Geometry: final body of the model. Coordinates: model frame, mm. A direction names the side the tool comes from. Give positions to 0.01 mm unless a question says otherwise; leave off trailing zeros. Write each loop counter-clockwise with the first axis right and the second up, starting at its lowest first coordinate (ties: lowest second). Pieces come first, ordered by that corner, then holes.
Q1. Section A-A (y = 38.5). Return the cut outline in (x, z), plus the area to 3 significant figures.
Q2. Section D-D (x = 96). Return the cut outline in (y, z), plus the area to 3 significant figures.
Q3. Section C-C (z = 14.75). Return the cut outline in (x, y), plus the area to 3 significant figures.
Q4. Mould query, pull axis X, two halves, no side actions, for faces 1 (the cylindrical face through (114, 4.57, 14.62)), 2 (the flat face through (1, 34, 7)). Classes: +X half, -X half, draft (parallel to the pull), parting line (faces both ways), or undercut.
Q5. Line query: line 1 (Y direction, x = 57, z = 6.2); line 2 (X direction, y = 53.5, z = 17.5); line 3 (Y direction, x = 19.5, z = 6.25). Output: solid intervals per line, ascending.
Q6. Section B-B (x = 115.5). Return the cut outline in (y, z).
Q7. Reachability of faces 3 (the cylindrical face through (5.306, 76.765, 14.619)), 4 (the flat face through (3, 74, 6)), 5 (the flat face through (57, 53, 3)) from +Z, -Z, +X, -X, +Y, -Y: full face, straight path, thin tool, end or side. Return the list, or none.
Q8. Pin query (flat end, axial travel): pin 1 Ø5 at (x, y) = (89, 65.5) entering from +Z. Return the tip coordinate at first contact, or that it passes through.
from build123d import *

# Parameters (mm, degrees)
ESQUISSE1_W             = 120
ESQUISSE1_H             = 80
BOSS_EXTRU_1_DEPTH      = 3
ESQUISSE4_W             = 120
ESQUISSE4_H             = 80
ESQUISSE4_W_2           = 114
ESQUISSE4_H_2           = 74
BOSS_EXTRU_3_DEPTH      = 20
CONG_1_R                = 15
ESQUISSE5_R             = 1.5
ENL_V_MAT_EXTRU_1_DEPTH = 147.044513762
ESQUISSE7_R             = 3
ENL_V_MAT_EXTRU_3_DEPTH = 6
ESQUISSE8_W             = 6
ESQUISSE8_H             = 6
ESQUISSE8_R             = 1.5
BOSS_EXTRU_4_DEPTH      = 5
ENL_V_MAT_EXTRU_4_REACH = 148.045
ESQUISSE9_W             = 7
ESQUISSE9_H             = 12
CONG_3_R                = 1


with BuildPart() as part:
    # Esquisse1 → Boss.-Extru.1 (new body)
    with BuildSketch(Plane.XY):
        with Locations((60, 40)):
            Rectangle(ESQUISSE1_W, ESQUISSE1_H)
    extrude(amount=BOSS_EXTRU_1_DEPTH)

    # Esquisse4 → Boss.-Extru.3 (add)
    with BuildSketch(Plane.XY.offset(3)):
        with Locations((60, 40)):
            Rectangle(ESQUISSE4_W, ESQUISSE4_H)
        with Locations((60, 40)):
            Rectangle(ESQUISSE4_W_2, ESQUISSE4_H_2, mode=Mode.SUBTRACT)
    extrude(amount=BOSS_EXTRU_3_DEPTH)

    # Congé1
    cong_1_edges = [part.edges().sort_by_distance(p)[0] for p in [
        (3, 3, 13),
        (117, 3, 13),
        (117, 77, 13),
        (3, 77, 13),
    ]]
    fillet(cong_1_edges, radius=CONG_1_R)

    # Esquisse5 → Enlèv. mat.-Extru.1 (cut, through all)
    with BuildSketch(Plane.XY.offset(23)):
        with Locations((4.5, 75.5)):
            Circle(ESQUISSE5_R)
        with Locations((115.5, 75.5)):
            Circle(ESQUISSE5_R)
        with Locations((115.5, 4.5)):
            Circle(ESQUISSE5_R)
        with Locations((4.5, 4.5)):
            Circle(ESQUISSE5_R)
    extrude(amount=-ENL_V_MAT_EXTRU_1_DEPTH, mode=Mode.SUBTRACT)

    # Esquisse7 → Enlèv. mat.-Extru.3 (cut)
    with BuildSketch(Plane(origin=(0, 0, 0), x_dir=(-1, 0, 0), z_dir=(0, 0, -1))):
        with Locations((-115.5, 75.5)):
            Circle(ESQUISSE7_R)
        with Locations((-4.5, 75.5)):
            Circle(ESQUISSE7_R)
        with Locations((-4.5, 4.5)):
            Circle(ESQUISSE7_R)
        with Locations((-115.5, 4.5)):
            Circle(ESQUISSE7_R)
    extrude(amount=-ENL_V_MAT_EXTRU_3_DEPTH, mode=Mode.SUBTRACT)

    # Esquisse8 → Boss.-Extru.4 (add)
    # profile 1 of 4: a face of its own
    with BuildSketch(Plane.XY.offset(3)):
        with Locations((6, 52.5)):
            Rectangle(ESQUISSE8_W, ESQUISSE8_H)
        with Locations((6, 52.5)):
            Circle(ESQUISSE8_R, mode=Mode.SUBTRACT)
    # profile 2 of 4: a face of its own
    with BuildSketch(Plane.XY.offset(3)):
        with Locations((57, 52.5)):
            Rectangle(ESQUISSE8_W, ESQUISSE8_H)
        with Locations((57, 52.5)):
            Circle(ESQUISSE8_R, mode=Mode.SUBTRACT)
    # profile 3 of 4: a face of its own
    with BuildSketch(Plane.XY.offset(3)):
        with Locations((57, 27.5)):
            Rectangle(ESQUISSE8_W, ESQUISSE8_H)
        with Locations((57, 27.5)):
            Circle(ESQUISSE8_R, mode=Mode.SUBTRACT)
    # profile 4 of 4: a face of its own
    with BuildSketch(Plane.XY.offset(3)):
        with Locations((6, 27.5)):
            Rectangle(ESQUISSE8_W, ESQUISSE8_H)
        with Locations((6, 27.5)):
            Circle(ESQUISSE8_R, mode=Mode.SUBTRACT)
    extrude(amount=BOSS_EXTRU_4_DEPTH)

    # Esquisse9 → Enlèv. mat.-Extru.4 (cut, up to next)
    with BuildSketch(Plane.ZY, mode=Mode.PRIVATE) as enl_v_mat_extru_4_sk1:
        with Locations((7, 40)):
            Rectangle(ESQUISSE9_W, ESQUISSE9_H)
    enl_v_mat_extru_4_tool1 = extrude(enl_v_mat_extru_4_sk1.sketch, amount=-ENL_V_MAT_EXTRU_4_REACH, mode=Mode.PRIVATE) & part.part
    add(enl_v_mat_extru_4_tool1.solids().sort_by_distance((0, 40, 7))[0], mode=Mode.SUBTRACT)

    # Congé3
    cong_3_edges = [part.edges().sort_by_distance(p)[0] for p in [
        (60, 80, 0),
        (120, 40, 0),
        (60, 0, 0),
        (0, 80, 11.5),
        (120, 80, 11.5),
        (120, 0, 11.5),
        (0, 0, 11.5),
    ]]
    fillet(cong_3_edges, radius=CONG_3_R)


solid = part.part
Computed:
1. outline: (0, 0) - (119, 0) arc R1 ccw to (120, 1) - (120, 23) - (117, 23) - (117, 3) - (3, 3) - (3, 3.5) - (0, 3.5) - close; (0, 10.5) - (3, 10.5) - (3, 23) - (0, 23) - close
1. area: 459 mm2
2. outline: (0, 1) arc R1 ccw to (1, 0) - (79, 0) arc R1 ccw to (80, 1) - (80, 23) - (77, 23) - (77, 3) - (3, 3) - (3, 23) - (0, 23) - close
2. area: 360 mm2
3. outline: (0, 1) arc R1 ccw to (1, 0) - (119, 0) arc R1 ccw to (120, 1) - (120, 79) arc R1 ccw to (119, 80) - (1, 80) arc R1 ccw to (0, 79) - close; hole circle Ø3 at (4.5, 4.5); hole (3, 18) arc R15 ccw to (18, 3) - (102, 3) arc R15 ccw to (117, 18) - (117, 62) arc R15 ccw to (102, 77) - (18, 77) arc R15 ccw to (3, 62) - close; hole circle Ø3 at (4.5, 75.5); hole circle Ø3 at (115.5, 4.5); hole circle Ø3 at (115.5, 75.5)
3. area: 1,330 mm2
4. face 1: undercut
4. face 2: draft
5. line 1: y = 0 to 3, 24.5 to 26, 29 to 30.5, 49.5 to 51, 54 to 55.5, 77 to 80
5. line 2: x = 0 to 3, 117 to 120
5. line 3: y = 0 to 3, 77 to 80
6. outline: (0, 1) arc R1 ccw to (1, 0) - (1.5, 0) - (1.5, 6) - (3, 6) - (3, 23) - (0, 23) - close; (6, 6) - (7.5, 6) - (7.5, 0) - (72.5, 0) - (72.5, 6) - (74, 6) - (74, 23) - (68.54, 23) - (68.54, 3) - (11.46, 3) - (11.46, 23) - (6, 23) - close; (77, 6) - (78.5, 6) - (78.5, 0) - (79, 0) arc R1 ccw to (80, 1) - (80, 23) - (77, 23) - close
7. face 3: +Z, -Z
7. face 4: -Z
7. face 5: +Z
8. pin 1: stops at z = 3
